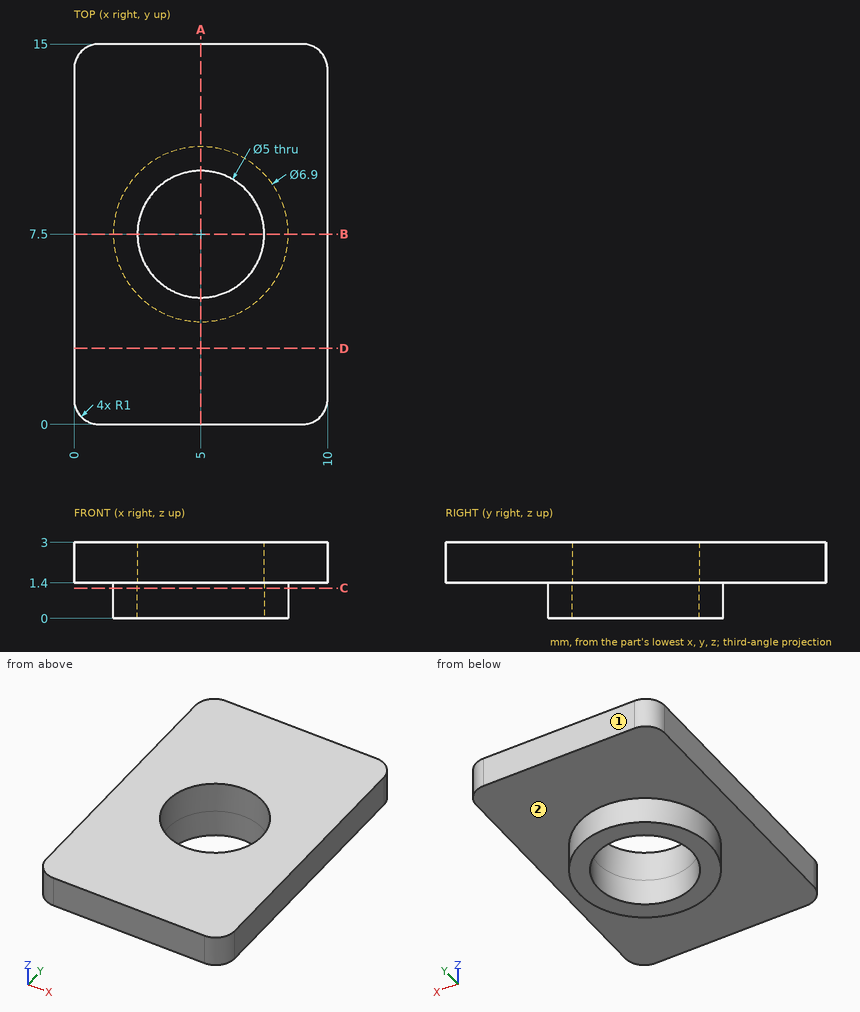
Can you work these out from the drawing? Everything is in mm from the part's minimum corner. A direction names the side the tool comes from. Round coordinates to 2 decimals unless told otherwise and drop trailing zeros. Write each loop counter-clockwise with the first axis right and the second up, starting at its lowest first coordinate (ties: lowest second). Pieces come first, ordered by that corner, then holes. Notation, with made-up numbers: M -16.75,63.5 L 31.25,63.5 A31 ccw 31.25,92.5 Z; hole C 43.5,-13.5 d1. An arc over 180 degrees is marked long. Use a Markdown table: item, result.
Item 1: I want a section at D-D (y = 3). List the corners of the cut face in (x, z) for me, and give its area (3 significant figures).
Found:
| item | result |
|---|---|
| outline | M 0,1.4 L 10,1.4 L 10,3 L 0,3 Z |
| area | 16.0 mm2 |
Item 2: If I drill on line 1 along Y through (x, z) = (5, 0.4); line 2 along Z through (x, y) = (8.5, 13); line 3 along X through (y, z) = (9.5, 2.05), over which ranges is the centre line in solid material (lowest first)? Write a range as [from, to].
Found:
| item | result |
|---|---|
| line 1 | y = [4.05, 5], [10, 10.95] |
| line 2 | z = [1.4, 3] |
| line 3 | x = [0, 3.5], [6.5, 10] |
Item 3: I want a section at C-C (z = 1.2). List the corners of the cut face in (x, y) for me.
Found:
| item | result |
|---|---|
| outline | C 5,7.5 d6.9; hole C 5,7.5 d5 |
Item 4: I want a section at A-A (x = 5). List the corners of the cut face in (y, z) for me, and give its area (3 significant figures).
Found:
| item | result |
|---|---|
| outline | M 0,1.4 L 4.05,1.4 L 4.05,0 L 5,0 L 5,3 L 0,3 Z; M 10,0 L 10.95,0 L 10.95,1.4 L 15,1.4 L 15,3 L 10,3 Z |
| area | 18.7 mm2 |
Item 5: Which directions (+Z, -Z, +X, -X, +Y, -Y) give clear straight access to the entire face, cutting with the end or side of a thin tool? Please do the marked faces 1 and 2.
Found:
| item | result |
|---|---|
| face 1 | +Z, -Z, +X, -X, +Y |
| face 2 | -Z |
Item 6: I want a section at B-B (y = 7.5). List the corners of the cut face in (x, z) for me, and give its area (3 significant figures).
Found:
| item | result |
|---|---|
| outline | M 0,1.4 L 1.55,1.4 L 1.55,0 L 2.5,0 L 2.5,3 L 0,3 Z; M 7.5,0 L 8.45,0 L 8.45,1.4 L 10,1.4 L 10,3 L 7.5,3 Z |
| area | 10.7 mm2 |
